Autodesk Inventor part; units mm, degrees
ref_plane "YZ Plane" through (0, 0, 0) normal (1, 0, 0) x (0, 1, 0)
ref_plane "XZ Plane" through (0, 0, 0) normal (0, 1, 0) x (-1, 0, 0)
ref_plane "XY Plane" through (0, 0, 0) normal (0, 0, 1) x (1, 0, 0)
sketch "Sketch1" plane through (0, 0, 0) normal (0, 1, 0) x (-1, 0, 0)
  line L0 (15, 32.5) -> (-15, 32.5)
  line L1 (-15, 32.5) -> (-15, -32.5)
  line L2 (-15, -32.5) -> (15, -32.5)
  line L3 (15, -32.5) -> (15, 32.5)
  line L4 (15, 32.5) -> (-15, -32.5) construction
  line L5 (-15, 32.5) -> (15, -32.5) construction
  line L6 (11.5, 29) -> (-11.5, 29) construction
  line L7 (-11.5, 29) -> (-11.5, -29) construction
  line L8 (-11.5, -29) -> (11.5, -29) construction
  line L9 (11.5, -29) -> (11.5, 29) construction
  line L10 (11.5, 29) -> (-11.5, -29) construction
  line L11 (-11.5, 29) -> (11.5, -29) construction
  circle A0 centre (11.5, 29) radius 1.25
  circle A1 centre (11.5, -29) radius 1.25
  circle A2 centre (-11.5, -29) radius 1.25
  circle A3 centre (-11.5, 29) radius 1.25
  point P0 (0, 0)
  dimension "d0" = 30
  dimension "d1" = 65
  dimension "d2" = 23
  dimension "d3" = 58
  dimension "d4" = 2.5
  dimension "d5" = 2.5
  dimension "d6" = 2.5
  dimension "d7" = 2.5
extrude "Extrusion1" add sketch "Sketch1" along normal blind 1
fillet "Fillet1" radius 3 4 edges at (-15, 0.5, 32.5) (15, 0.5, 32.5) (15, 0.5, -32.5) (-15, 0.5, -32.5)
sketch "Sketch2" plane through (0, 1, 0) normal (0, 1, 0) x (1, 0, 0)
  line L0 (-14.25, -25.5) -> (-8.75, -25.5)
  line L1 (-8.75, -25.5) -> (-8.75, 25.5)
  line L2 (-8.75, 25.5) -> (-14.25, 25.5)
  line L3 (-14.25, 25.5) -> (-14.25, -25.5)
  line L4 (-14.25, -25.5) -> (-8.75, 25.5) construction
  line L5 (-8.75, -25.5) -> (-14.25, 25.5) construction
  line L6 (-15, 29.5) -> (-15, -29.5)
  point P0 (0, 0)
  point P1 (-11.5, 0)
  dimension "d11" = 5.5
  dimension "d12" = 51
  dimension "d13" = 3.5
extrude "Extrusion2" add sketch "Sketch2" along normal blind 10 and the other way blind 3
properties part number "raspberry"
Input: part model. Units: mm. Frame: model coordinates. A direction names the side the tool comes from. Round coordinates to 2 decimals unless told otherwise and drop trailing zeros. Loops run counter-clockwise (first coordinate to the right, second up) from the corner with the lowest first, then second, coordinate; pieces in that order, holes last. Notation, with made-up numbers: (3, 60) -> (36, 60) arc R21 ccw to (36, 85) -> close; hole circle Ø3 at (88, -35). An arc over 180 degrees is marked (long way). Use one line per item in the form item = value. Start each with the question number.
Item 1: Material intervals for L1, parallel to Z at x = -11.5, y = 0.5; L2, parallel to Z at x = -13.25, y = 7.5; L3, parallel to X at y = 4, z = -18.5, sorted ascending. Write a range as from..to.
Item 2: Section query C-C on y = 3.25. Return the cut outline in (x, z), then the cut area to 4 significant figures.
Item 3: Set-up query: faces 1 (the face through (-11, 6, -25.5)), 2 (the face through (-12, 6, 25.5)), 3 (the face through (-14.25, -1, 0)). Return all of +Z, -Z, +X, -X, +Y, -Y with unobstructed straight access to the full face (end or side cutting, diameter ignored); none if empty.
Item 4: Section query A-A on z = -20.5. Return the cut outline in (x, y), then the cut area to 3 significant figures.
Item 5: Section query B-B on x = -1.25. Return the cut outline in (y, z).
Item 6: Contact query for flat-ended pins moving along their axis: pin 1 Ø3 at (y, z) = (8.5, 4.5) entering from -X; pin 2 Ø10 at (x, z) = (4.5, 0.5) entering from -Y; pin 3 Ø3 at (x, z) = (11.5, 29) entering from +Y; pin 4 Ø1.5 at (y, z) = (1.5, 18.5) entering from +X. Output: stop coordinate, or through.
Ans:
q1.L1 = -32.5..-30.25, -27.75..27.75, 30.25..32.5
q1.L2 = -25.5..25.5
q1.L3 = -14.25..-8.75
q2.outline = (-14.25, -25.5) -> (-8.75, -25.5) -> (-8.75, 25.5) -> (-14.25, 25.5) -> close
q2.area = 280.5 mm^2
q3.face_1 = -Z, +X, -X, +Y
q3.face_2 = +Z, +X, -X, +Y
q3.face_3 = +Z, -Z, -X, -Y
q4.outline = (-15, 0) -> (-14.25, 0) -> (-14.25, -2) -> (-8.75, -2) -> (-8.75, 0) -> (15, 0) -> (15, 1) -> (-8.75, 1) -> (-8.75, 11) -> (-14.25, 11) -> (-14.25, 1) -> (-15, 1) -> close
q4.area = 96.0 mm^2
q5.outline = (0, -32.5) -> (1, -32.5) -> (1, 32.5) -> (0, 32.5) -> close
q6.pin_1 = -14.25
q6.pin_2 = 0
q6.pin_3 = 1
q6.pin_4 = 15
